The listing builds one solid part. Answer for the finished solid, in the listing's coordinates (mm). Face numbers are marked on the shaded views. A direction names the side the tool comes from. Give positions to 0.01 mm unless a question says otherwise; leave off trailing zeros. Write each loop counter-clockwise with the first axis right and the second up, starting at its lowest first coordinate (ties: lowest second). Pieces come first, ordered by that corner, then holes. Notation, with made-up numbers: (-11, 66.25) - (29, 66.25) arc R14 cw to (29, 92.25) - close; hole circle Ø11 at (-25, -8.75). An arc over 180 degrees is marked (long way). One line per question, with ' | ' between items. Start each with the question number.
1. A cutting plane is placed at B-B (y = 17.5). Determine the outline of the cut face in (x, z), then the cut area to 3 significant figures.
2. Given P1, Ø3, axis at x = 29.5, z = -5, coming from the +Y side; P2, Ø6.5, axis at x = 15.5, z = 2.5, coming from the -Y side; P3, Ø10, axis at x = 15, y = -31, coming from the +Z side; P4, Ø3, axis at x = 22.705, y = 2.935, coming from the +Z side, each flat-ended and moving along its own axis, determine where each tip first touches the part or whether it passes through.
3. A cutting plane is placed at C-C (z = 4.5). Determine the outline of the cut face in (x, y) (3 decimals), then the cut area to 3 significant figures.
4. The mould has two halves that part along Z. Classify the marked faces 1, 2 and 3: +Z half, -Z half, draft (parallel to the pull), parting line (faces both ways), or undercut.
5. A cutting plane is placed at D-D (x = 16.23). Determine the outline of the cut face in (y, z).
6. For the marked faces 4, 5, 6, 7 and 8, determine the directions among +Z, -Z, +X, -X, +Y, -Y from which every point of the face is accessible in a straight line to the end or side of a thin tool.
7. A cutting plane is placed at A-A (x = 27). Determine the outline of the cut face in (y, z).
8. Find the intervals of material crossed by L1, parallel to Y at x = 16.23, z = 1.75; L2, parallel to Z at x = 28, y = -3.5; L3, parallel to Z at x = 23, y = 1.5, in increasing order. Write a range as from..to.
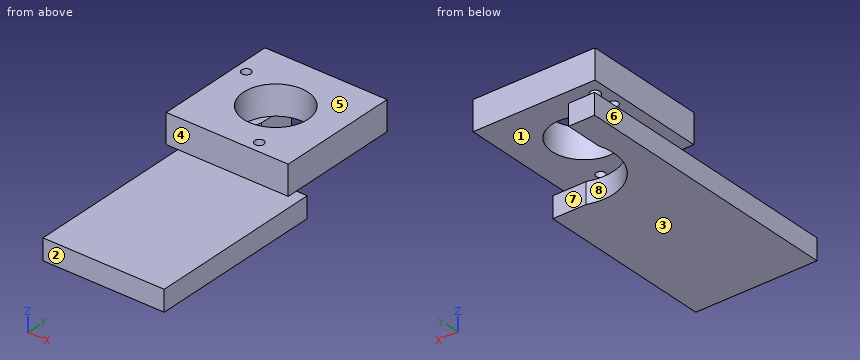
```python
from build123d import *

# Parameters (mm, degrees)
SKETCH1_W           = 32.86
SKETCH1_H           = 33.04
SKETCH1_R           = 8.68
SKETCH1_R_2         = 1.245
BOSS_EXTRUDE1_DEPTH = 7.95
SKETCH2_R           = 1.271766889
BOSS_EXTRUDE2_DEPTH = 3
BOSS_EXTRUDE3_DEPTH = 5.66


with BuildPart() as part:
    # Sketch1 → Boss-Extrude1 (new body)
    with BuildSketch(Plane.XY):
        with Locations((16.43, 16.52)):
            Rectangle(SKETCH1_W, SKETCH1_H)
        with Locations((16.23, 16.48)):
            Circle(SKETCH1_R, mode=Mode.SUBTRACT)
        with Locations((2.935, 23.145)):
            Circle(SKETCH1_R_2, mode=Mode.SUBTRACT)
        with Locations((22.705, 2.935)):
            Circle(SKETCH1_R_2, mode=Mode.SUBTRACT)
    extrude(amount=BOSS_EXTRUDE1_DEPTH)

    # Sketch2 → Boss-Extrude2 (add)
    with BuildSketch(Plane(origin=(0, 0, 0), x_dir=(-1, 0, 0), z_dir=(0, 0, -1))):
        with Locations((-3.305838701, 28.863410922)):
            Circle(SKETCH2_R)
    extrude(amount=BOSS_EXTRUDE2_DEPTH)

    # Sketch3 → Boss-Extrude3 (add)
    with BuildSketch(Plane(origin=(0, 0, -3), x_dir=(-1, 0, 0), z_dir=(0, 0, -1))):
        with BuildLine():
            Line((-0.1, 33.04), (-7.1, 33.04))
            Line((-7.1, 33.04), (-7.1, 23.04))
            ThreePointArc((-7.1, 23.04), (-10.265055125, 9.570142898), (-23.75, 6.47))
            Line((-23.75, 6.47), (-32.75, 6.47))
            Line((-32.75, 6.47), (-32.75, -41.35))
            Line((-32.75, -41.35), (-0.1, -41.35))
            Line((-0.1, -41.35), (-0.1, 33.04))
        make_face()
    extrude(amount=BOSS_EXTRUDE3_DEPTH)


solid = part.part
```
Determined:
1) outline: (0, 0) - (7.61, 0) - (7.61, 7.95) - (0, 7.95) - close; (0.1, -8.66) - (6.48, -8.66) - (6.48, -3) - (0.1, -3) - close; (24.85, 0) - (32.86, 0) - (32.86, 7.95) - (24.85, 7.95) - close | area: 160 mm2
2) P1: y = 6.47 | P2: y = 0 | P3: z = -3 | P4: z = 7.95
3) outline: (0, 0) - (32.86, 0) - (32.86, 33.04) - (0, 33.04) - close; hole circle Ø2.49 at (2.935, 23.145); hole circle Ø17.36 at (16.23, 16.48); hole circle Ø2.49 at (22.705, 2.935) | area: 839 mm2
4) face 1: undercut | face 2: draft | face 3: -Z half
5) outline: (-41.35, -8.66) - (6.17, -8.66) - (6.17, -3) - (-41.35, -3) - close; (0, 0) - (7.8, 0) - (7.8, 7.95) - (0, 7.95) - close; (25.16, 0) - (33.04, 0) - (33.04, 7.95) - (25.16, 7.95) - close
6) face 4: +Z, +X, -X, -Y | face 5: +Z, +X, -X, +Y, -Y | face 6: -Z, -X, +Y, -Y | face 7: -Z, +X, +Y | face 8: -Z
7) outline: (-41.35, -8.66) - (6.47, -8.66) - (6.47, -3) - (-41.35, -3) - close; (0, 0) - (33.04, 0) - (33.04, 7.95) - (0, 7.95) - close
8) L1: 0..7.8, 25.16..33.04 | L2: -8.66..-3 | L3: -8.66..-3, 0..7.95
